Source: CAD feature listing. Evaluate the final solid. Frame: model axes, mm. Face numbers are marked on the shaded views. A direction names the side the tool comes from. Coordinates: 2 decimals unless noted, no trailing zeros. Order: outer loops, then holes, each group sorted by start corner. A loop starts at its lowest first (then second) coordinate and runs counter-clockwise, first axis right, second up. Notation, with made-up numbers: (80.25, 36) - (103.25, 36) arc R28 ccw to (103.25, 62) - close; hole circle Ø7 at (88.5, -4). An arc over 180 degrees is marked (long way). One line per question, with ' | ' between items. Start each with the question number.
(1) Access query for the marked faces 4, 5, 6, 7 and 8. Directions: +Z, -Z, +X, -X, +Y, -Y. A direction counts if a zero-diameter tool reaches every point of the face in a straight line with its end or side. Return the directions, or none.
(2) Section A-A (z = 8.25). Return the cut outline in (x, y), then the cut area to 3 significant figures.
(3) Section B-B (y = 0). Return the cut outline in (x, z), then the cut area to 3 significant figures.
(4) Draft query along X for the marked faces 1, 2 and 3. Return one class per face: +X half, -X half, draft (parallel to the pull), parting line (faces both ways), or undercut.
(5) Contact query for flat-ended pins moving along their axis: P1, Ø2.5, axis at y = 24, z = 7, coming from the -X side; P2, Ø1.2, axis at x = -0.5, z = 5.5, coming from the -Y side; P3, Ø5, axis at y = -2.5, z = 4.5, coming from the +X side; P4, Ø5, axis at x = -4, y = -1.5, coming from the -Z side. Output: stop coordinate, or through.
(6) Section D-D (x = 18.5). Return the cut outline in (y, z).
(7) Line query: line 1 along Y through (x, z) = (0, 3.1); line 2 along Y through (x, z) = (1.5, 7.75). Output: solid intervals per line, ascending.
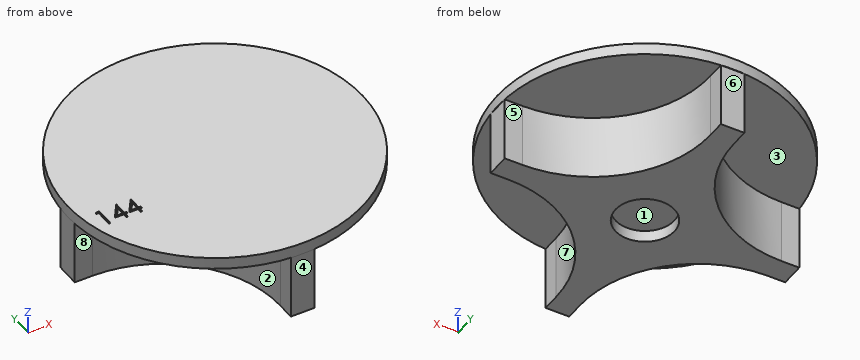
from build123d import *

# Parameters (mm, degrees)
BOSS_EXTRUDE1_START = 2
BOSS_EXTRUDE1_DEPTH = 13
SKETCH7_R           = 25.106657787
BOSS_EXTRUDE3_DEPTH = 2
SKETCH8_R           = 5
CUT_EXTRUDE2_DEPTH  = 4
CUT_EXTRUDE3_DEPTH  = 0.3


with BuildPart() as part:
    # Sketch4 → Boss-Extrude1 (new body)
    with BuildSketch(Plane.XY.offset(BOSS_EXTRUDE1_START)):
        with BuildLine():
            Line((-25, 2), (-25, 0))
            Line((-25, 0), (25, 0))
            Line((25, 0), (25, 2))
            Line((25, 2), (22, 2))
            ThreePointArc((22, 2), (7.857864376, 7.857864376), (2, 22))
            Line((2, 22), (2, 25))
            Line((2, 25), (-2, 25))
            Line((-2, 25), (-2, 22))
            ThreePointArc((-2, 22), (-7.857864376, 7.857864376), (-22, 2))
            Line((-22, 2), (-25, 2))
        make_face()
        with BuildLine():
            Line((25, 0), (-25, 0))
            Line((-25, 0), (-25, -2))
            Line((-25, -2), (-22, -2))
            ThreePointArc((-22, -2), (-7.857864376, -7.857864376), (-2, -22))
            Line((-2, -22), (-2, -25))
            Line((-2, -25), (2, -25))
            Line((2, -25), (2, -22))
            ThreePointArc((2, -22), (7.857864376, -7.857864376), (22, -2))
            Line((22, -2), (25, -2))
            Line((25, -2), (25, 0))
        make_face()
    extrude(amount=BOSS_EXTRUDE1_DEPTH)

    # Sketch7 → Boss-Extrude3 (add)
    with BuildSketch(Plane(origin=(0, 0, 15), x_dir=(-1, 0, 0), z_dir=(0, 0, -1))):
        Circle(SKETCH7_R)
    extrude(amount=BOSS_EXTRUDE3_DEPTH)

    # Sketch8 → Cut-Extrude2 (cut)
    with BuildSketch(Plane.XY):
        Circle(SKETCH8_R)
    extrude(amount=CUT_EXTRUDE2_DEPTH, mode=Mode.SUBTRACT)

    # Sketch11 → Cut-Extrude3 (cut)
    # profile 1 of 3: a face of its own
    with BuildSketch(Plane.XY.offset(15)):
        Polygon((-22.334208893, -3.554058613), (-21.747164623, -3.554058613), (-21.747164623, -6.729058613), (-22.03210052, -6.729058613), (-22.03210052, -3.879699638), (-22.520562059, -3.879699638), align=None)
    # profile 2 of 3: a face of its own
    with BuildSketch(Plane.XY.offset(15)):
        Polygon((-18.833567868, -3.472648356), (-18.775690264, -3.472648356), (-18.775690264, -5.670725279), (-18.40934411, -5.670725279), (-18.40934411, -5.996366305), (-18.775690264, -5.996366305), (-18.775690264, -6.729058613), (-19.060626161, -6.729058613), (-19.060626161, -5.996366305), (-20.566715905, -5.996366305), align=None)
        Polygon((-19.060626161, -5.670725279), (-19.060626161, -4.291839062), (-20.007020392, -5.670725279), align=None, mode=Mode.SUBTRACT)
    # profile 3 of 3: a face of its own
    with BuildSketch(Plane.XY.offset(15)):
        Polygon((-16.391260175, -3.472648356), (-16.333382571, -3.472648356), (-16.333382571, -5.670725279), (-15.967036417, -5.670725279), (-15.967036417, -5.996366305), (-16.333382571, -5.996366305), (-16.333382571, -6.729058613), (-16.618318469, -6.729058613), (-16.618318469, -5.996366305), (-18.124408212, -5.996366305), align=None)
        Polygon((-16.618318469, -5.670725279), (-16.618318469, -4.291839062), (-17.5647127, -5.670725279), align=None, mode=Mode.SUBTRACT)
    extrude(amount=-CUT_EXTRUDE3_DEPTH, mode=Mode.SUBTRACT)


solid = part.part
Response values:
1) face 4: -Z, +X, -X, -Y | face 5: -Z, +X, +Y | face 6: -Z, +X, -X, +Y | face 7: -Z, +X, -Y | face 8: -Z, -X, -Y
2) outline: (-25, -2) - (-22, -2) arc R20 cw to (-2, -22) - (-2, -25) - (2, -25) - (2, -22) arc R20 cw to (22, -2) - (25, -2) - (25, 2) - (22, 2) arc R20 cw to (2, 22) - (2, 25) - (-2, 25) - (-2, 22) arc R20 cw to (-22, 2) - (-25, 2) - close | area: 727 mm²
3) outline: (-25.11, 13) - (-25, 13) - (-25, 2) - (-5, 2) - (-5, 4) - (5, 4) - (5, 2) - (25, 2) - (25, 13) - (25.11, 13) - (25.11, 15) - (-25.11, 15) - close | area: 630 mm²
4) face 1: undercut | face 2: -X half | face 3: draft
5) P1: stops at x = -2 | P2: stops at y = -25 | P3: stops at x = 25 | P4: stops at z = 2
6) outline: (-16.97, 13) - (-2.31, 13) - (-2.31, 2) - (2.31, 2) - (2.31, 13) - (16.97, 13) - (16.97, 15) - (-16.97, 15) - close
7) line 1: y = -25 to -5, 5 to 25 | line 2: y = -25 to 25
